Here's how the part is built. I have some questions about the finished solid (model axes, mm). Face numbers are marked on the shaded views. A direction names the side the tool comes from. Coordinates: 2 decimals unless noted, no trailing zeros. Order: outer loops, then holes, each group sorted by start corner. A loop starts at its lowest first (then second) coordinate and runs counter-clockwise, first axis right, second up. Notation, with made-up numbers: (-6, 66) - (27, 66) arc R35 cw to (27, 105) - close; hole circle Ø6 at (-5, 68). An arc over 180 degrees is marked (long way). Answer as CSV lines item,"result". Start each with the question number.
Q1. I need wall thicknesses on line 1 (Z direction, x = 21.5, y = -44.5); line 2 (Y direction, x = 25, z = 18.25); line 3 (Z direction, x = 5.5, y = 15). Which ranges of each line are inside material? Lowest first, please.
Q2. Suppose I cut it at D-D (y = -40.5). Please give me the cut outline in (x, z).
Q3. Suppose I cut it at C-C (z = 15). Please give me the cut outline in (x, y), then the cut area to 3 significant figures.
Q4. For the marked faces 1 and 2, which set-ups out of +Z, -Z, +X, -X, +Y, -Y let a thin tool reach every point of the face, with its end or its side?
Q5. Suppose I cut it at A-A (y = -12.5). Please give me the cut outline in (x, z).
Q6. For pin 1 Ø5 at (x, y) = (7.5, -12) entering from +Z; pin 2 Ø1 at (x, z) = (-19.5, 15.5) entering from -Y; pin 3 Ø12 at (x, y) = (-10.5, -19) entering from -Z, each with a flat end and sliding along its axis, tell me the tip position at first contact or that it passes through.
Q7. Suppose I cut it at B-B (x = -7). Please give me the cut outline in (y, z).
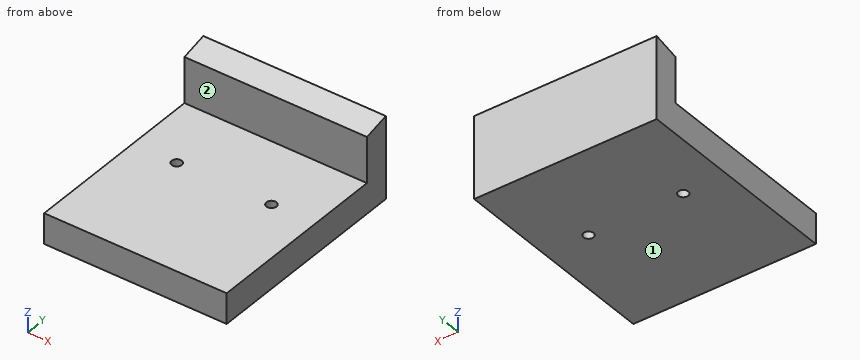
from build123d import *

# Parameters (mm, degrees)
ESQUISSE1_W           = 60
ESQUISSE1_H           = 70
BOSS_EXTRU_1_DEPTH    = 10
BOSS_EXTRU_2_DEPTH    = 60
TROU_TARAUD_M41_D     = 3.3
TROU_TARAUD_M41_DEPTH = 11.5
TROU_TARAUD_M41_TIP   = 0.991420021


with BuildPart() as part:
    # Esquisse1 → Boss.-Extru.1 (new body)
    with BuildSketch(Plane.XY):
        with Locations((3.076402568, -15.684931507)):
            Rectangle(ESQUISSE1_W, ESQUISSE1_H)
    extrude(amount=BOSS_EXTRU_1_DEPTH)

    # Esquisse2 → Boss.-Extru.2 (add)
    with BuildSketch(Plane(origin=(33.076402568, 0, 0), x_dir=(0, 0, -1), z_dir=(1, 0, 0))):
        Polygon((-27, 19.315068493), (-25, 11.018826061), (-10, 11.018826061), (-10, 19.315068493), align=None)
    extrude(amount=-BOSS_EXTRU_2_DEPTH)

    # Trou taraudé M41
    with Locations(Plane(origin=(18.651402568, -11.684931507, 0), x_dir=(-1, 0, 0), z_dir=(0, 0, -1))):
        with Locations((0, 0), (31.15, 0)):
            Hole(TROU_TARAUD_M41_D / 2, depth=TROU_TARAUD_M41_DEPTH)
            with Locations((0, 0, -(TROU_TARAUD_M41_DEPTH + TROU_TARAUD_M41_TIP / 2))):  # 118° drill point
                Cone(0, TROU_TARAUD_M41_D / 2, TROU_TARAUD_M41_TIP, mode=Mode.SUBTRACT)


solid = part.part
Here are the results:
1,line 1,"z = 0 to 10"
1,line 2,"y = 11.02 to 19.32"
1,line 3,"z = 0 to 25.96"
2,outline,"(-26.92, 0) - (33.08, 0) - (33.08, 10) - (-26.92, 10) - close"
3,outline,"(-26.92, 11.02) - (33.08, 11.02) - (33.08, 19.32) - (-26.92, 19.32) - close"
3,area,"498 mm²"
4,face 1,"-Z, +X, -X, +Y, -Y"
4,face 2,"+Z, +X, -X, -Y"
5,outline,"(-26.92, 0) - (-13.93, 0) - (-13.93, 10) - (-26.92, 10) - close; (-11.06, 0) - (17.22, 0) - (17.22, 10) - (-11.06, 10) - close; (20.09, 0) - (33.08, 0) - (33.08, 10) - (20.09, 10) - close"
6,pin 1,"stops at z = 10"
6,pin 2,"stops at y = 11.02"
6,pin 3,"stops at z = 0"
7,outline,"(-50.68, 0) - (19.32, 0) - (19.32, 27) - (11.02, 25) - (11.02, 10) - (-50.68, 10) - close"
